from build123d import *

# Parameters (mm, degrees)
F0_W          = 203.2
F0_H          = 127
F1_DEPTH      = 127
F3_DEPTH      = 76.2
F4_SIZE2      = 101.6
F4_SIZE       = 76.2
F5_R          = 5.08
F6_R          = 15.24
F7_DEPTH      = 25.4
F7_DEPTH_BACK = 76.2
F8_R          = 15.24
F9_DEPTH      = 254
F9_DEPTH_BACK = 254


with BuildPart() as f1:
    # F0 (on Front) → F1 (new body)
    with BuildSketch(Plane.XZ):
        Rectangle(F0_W, F0_H)
    extrude(amount=F1_DEPTH)

    # F2 (on face) → F3 (cut)
    with BuildSketch(Plane.XZ.offset(127)):
        Polygon((101.6, 63.5), (25.4, 63.5), (25.4, 0), (-41.4866656065, 0), (-41.4866656065, -63.5), (101.6, -63.5), align=None)
    extrude(amount=-F3_DEPTH, mode=Mode.SUBTRACT)

    # F4
    f4_edges = [f1.edges().sort_by_distance(p)[0] for p in [
        (101.6, -25.4, 63.5),
    ]]
    f4_side = f1.faces().sort_by_distance((-18.435484, -56.125806, 63.5))[0]
    chamfer(f4_edges, length=F4_SIZE, length2=F4_SIZE2, reference=f4_side)

    # F5
    f5_edges = [f1.edges().sort_by_distance(p)[0] for p in [
        (-38.1, -127, 63.5),
        (25.4, -88.9, 63.5),
        (25.4, -88.9, 0),
        (-8.043333, -127, 0),
        (-101.6, -63.5, 63.5),
        (-41.486666, -127, -31.75),
        (-41.486666, -88.9, -63.5),
        (-71.543333, -127, -63.5),
        (30.056667, -50.8, -63.5),
        (101.6, -25.4, -63.5),
        (101.6, -50.8, -50.8),
        (101.6, 0, -50.8),
        (101.6, -25.4, -38.1),
        (0, 0, -63.5),
        (-101.6, 0, 0),
        (-101.6, -63.5, -63.5),
        (25.4, -127, 31.75),
        (-101.6, -127, 0),
        (-38.1, 0, 63.5),
    ]]
    fillet(f5_edges, radius=F5_R)

    # F6 (on Front) → F7 (cut, two sides)
    with BuildSketch(Plane.XZ) as f7_sk:
        with Locations((19.9351496994, -20.7433328032)):
            Circle(F6_R)
    extrude(amount=-F7_DEPTH, mode=Mode.SUBTRACT)
    extrude(f7_sk.sketch, amount=F7_DEPTH_BACK, mode=Mode.SUBTRACT)

    # F8 (on face) → F9 (cut, two sides)
    with BuildSketch(Plane.XY.offset(63.5)) as f9_sk:
        with Locations((-75.8246555924, -103.2319366932)):
            Circle(F8_R)
    extrude(amount=-F9_DEPTH, mode=Mode.SUBTRACT)
    extrude(f9_sk.sketch, amount=F9_DEPTH_BACK, mode=Mode.SUBTRACT)


solid = f1.part
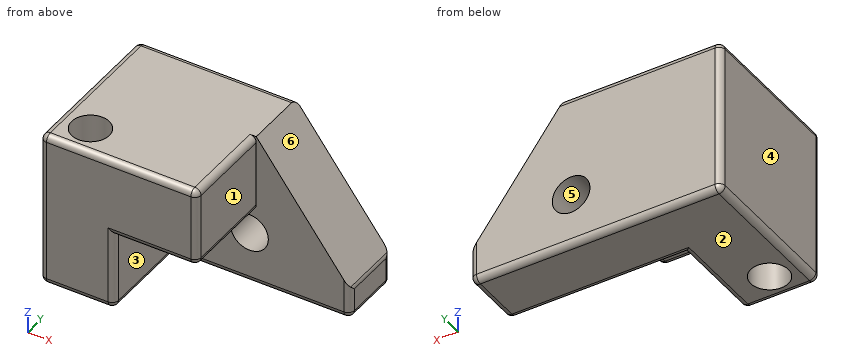
CAD build for the part. Positions are in the model's coordinates, mm. Face numbers are marked on the shaded views. A direction names the side the tool comes from. Give positions to 0.01 mm unless a question says otherwise; leave off trailing zeros. Write each loop counter-clockwise with the first axis right and the second up, starting at its lowest first coordinate (ties: lowest second). Pieces come first, ordered by that corner, then holes. Notation, with made-up numbers: (-4, 36.5) -> (4, 36.5) arc R21 ccw to (4, 68.5) -> close; hole circle Ø1 at (17.25, -40). An arc over 180 degrees is marked (long way). Return JSON: item names as keys, results as strings.
Item 1: Drop flat-ended pins along their axis: pin 1 (18.5 mm diameter, centred on x = -14, y = -97, fed in from -Z); pin 2 (5 mm diameter, centred on x = 48.5, z = -45.5, fed in from -Y); pin 3 (6 mm diameter, centred on y = -36.5, z = -10.5, fed in from +X). Give the stop position or say it passes through.
Answer below:
{"pin 1": "stops at z = 0", "pin 2": "stops at y = -50.8", "pin 3": "stops at x = 83.15"}
Item 2: Band-saw the part on C-C (z = 23). List the corners of the cut face in (x, y) (3 decimals).
Answer below:
{"outline": "(-101.6, -121.92) arc R5.08 ccw to (-96.52, -127) -> (20.32, -127) arc R5.08 ccw to (25.4, -121.92) -> (25.4, -50.8) -> (55.775, -50.8) -> (55.775, 0) -> (-96.52, 0) arc R5.08 ccw to (-101.6, -5.08) -> close; hole circle Ø30.48 at (-75.825, -103.232)"}
Item 3: Band-saw the part on B-B (y = -70). List the corners of the cut face in (x, z), then the cut area to 3 significant figures.
Answer below:
{"outline": "(-101.6, -58.42) arc R5.08 ccw to (-96.52, -63.5) -> (-46.57, -63.5) arc R5.08 ccw to (-41.49, -58.42) -> (-41.49, 0) -> (20.32, 0) arc R5.08 ccw to (25.4, 5.08) -> (25.4, 58.42) arc R5.08 ccw to (20.32, 63.5) -> (-96.52, 63.5) arc R5.08 ccw to (-101.6, 58.42) -> close", "area": "11,900 mm2"}
Item 4: Band-saw the part on D-D (x = -87.5). List the corners of the cut face in (y, z), then the cut area to 3 significant figures.
Answer below:
{"outline": "(-127, -58.42) arc R5.08 ccw to (-121.92, -63.5) -> (-113.03, -63.5) -> (-113.03, 63.5) -> (-121.92, 63.5) arc R5.08 ccw to (-127, 58.42) -> close; (-93.44, -63.5) -> (-5.08, -63.5) arc R5.08 ccw to (0, -58.42) -> (0, 58.42) arc R5.08 ccw to (-5.08, 63.5) -> (-93.44, 63.5) -> close", "area": "13,600 mm2"}
Item 5: Drill centre lines: probe 1 along X at (y, z) = (-47.5, -32) (3 decimals); probe 2 along X at (y, z) = (-86.5, -25.5); probe 3 along Y at (x, z) = (-65.5, -12). Where is each one in solid material? Low to high.
Answer below:
{"probe 1": "x = -101.6 to 9.662, 30.209 to 97.025", "probe 2": "x = -101.6 to -41.49", "probe 3": "y = -127 to -114.44, -92.02 to 0"}
Item 6: Two-plate mould, pull along X, no slides. Class the marked faces 4, 5 and 6: +X half, -X half, draft (parallel to the pull), parting line (faces both ways), or undercut.
Answer below:
{"face 4": "-X half", "face 5": "undercut", "face 6": "+X half"}
Item 7: Tool access for the marked faces 1, 2 and 3: list every direction of +Z, -Z, +X, -X, +Y, -Y with a clear straight run to the whole face (end or side of a thin tool).
Answer below:
{"face 1": "+Z, -Z, +X, -Y", "face 2": "-Z, +X, -X, +Y, -Y", "face 3": "-Z, +X, -Y"}
Item 8: Band-saw the part on A-A (x = -24). List the corners of the cut face in (y, z), then the cut area to 3 significant figures.
Answer below:
{"outline": "(-127, 5.08) arc R5.08 ccw to (-121.92, 0) -> (-50.8, 0) -> (-50.8, -58.42) arc R5.08 ccw to (-45.72, -63.5) -> (-5.08, -63.5) arc R5.08 ccw to (0, -58.42) -> (0, 58.42) arc R5.08 ccw to (-5.08, 63.5) -> (-121.92, 63.5) arc R5.08 ccw to (-127, 58.42) -> close", "area": "11,300 mm2"}
